```python
from build123d import *

# Parameters (mm, degrees)
SKETCH001_W     = 20
SKETCH001_H     = 84
PAD001_DEPTH    = 3
SKETCH002_W     = 20
SKETCH002_H     = 3
PAD002_DEPTH    = 10
SKETCH003_W     = 40
SKETCH003_H     = 8
SKETCH003_H_2   = 13
PAD003_DEPTH    = 3
FILLET_R        = 1
FILLET001_R     = 1
FILLET002_R     = 1
FILLET003_R     = 0.3
FILLET004_R     = 0.9
SKETCH009_W     = 10
SKETCH009_H     = 2
POCKET004_DEPTH = 5
POCKET005_DEPTH = 20


with BuildPart() as part:
    # Sketch001 → Pad001 (new body)
    with BuildSketch(Plane.XY):
        with Locations((0, -78.487457)):
            Rectangle(SKETCH001_W, SKETCH001_H)
    extrude(amount=PAD001_DEPTH)

    # Sketch002 → Pad002 (new body)
    with BuildSketch(Plane.XY.offset(3)):
        with Locations((0, -118.987457)):
            Rectangle(SKETCH002_W, SKETCH002_H)
        with Locations((0, -37.987457)):
            Rectangle(SKETCH002_W, SKETCH002_H)
    extrude(amount=PAD002_DEPTH)

    # Sketch003 → Pad003 (new body)
    with BuildSketch(Plane.XY.offset(13)):
        with Locations((0, -40.487457)):
            Rectangle(SKETCH003_W, SKETCH003_H)
        with Locations((0, -113.987457)):
            Rectangle(SKETCH003_W, SKETCH003_H_2)
    extrude(amount=PAD003_DEPTH)

    # Fillet
    fillet_edges = [part.edges().sort_by_distance(p)[0] for p in [
        (20, -113.987457, 16),
        (20, -113.987457, 13),
        (-20, -113.987457, 16),
        (0, -107.487457, 16),
        (0, -120.487457, 16),
        (-20, -113.987457, 13),
        (-15, -120.487457, 13),
        (15, -120.487457, 13),
    ]]
    fillet(fillet_edges, radius=FILLET_R)

    # Fillet001
    fillet001_edges = [part.edges().sort_by_distance(p)[0] for p in [
        (20, -40.487457, 16),
        (0, -44.487457, 16),
        (0, -36.487457, 16),
        (-20, -40.487457, 16),
        (-20, -40.487457, 13),
        (-15, -36.487457, 13),
        (15, -36.487457, 13),
        (20, -40.487457, 13),
        (0, -44.487457, 13),
    ]]
    fillet(fillet001_edges, radius=FILLET001_R)

    # Fillet002
    fillet002_edges = [part.edges().sort_by_distance(p)[0] for p in [
        (-10, -78.487457, 3),
        (-10, -117.487457, 8),
        (-10, -120.487457, 6.5),
        (-10, -78.487457, 0),
        (-10, -36.487457, 6.5),
        (10, -39.487457, 8),
        (10, -36.487457, 6.5),
        (10, -78.487457, 0),
        (10, -78.487457, 3),
        (10, -117.487457, 8),
        (10, -120.487457, 6.5),
    ]]
    fillet(fillet002_edges, radius=FILLET002_R)

    # Fillet003
    fillet003_edges = [part.edges().sort_by_distance(p)[0] for p in [
        (0, -39.487457, 3),
        (0, -117.487457, 3),
    ]]
    fillet(fillet003_edges, radius=FILLET003_R)

    # Fillet004
    fillet004_edges = [part.edges().sort_by_distance(p)[0] for p in [
        (0, -107.487457, 13),
    ]]
    fillet(fillet004_edges, radius=FILLET004_R)

    # Sketch009 → Pocket004 (cut)
    with BuildSketch(Plane(origin=(0, 0, 0), x_dir=(1, 0, 0), z_dir=(0, 0, -1))):
        with Locations((0, 40.487457)):
            Rectangle(SKETCH009_W, SKETCH009_H)
    extrude(amount=-POCKET004_DEPTH, mode=Mode.SUBTRACT)

    # Sketch012 → Pocket005 (cut)
    with BuildSketch(Plane(origin=(0, -36.487457, 0), x_dir=(-1, 0, 0), z_dir=(0, 1, 0))):
        with BuildLine():
            ThreePointArc((-4, 2), (-4.5, 1.5), (-4, 1))
            Line((-4, 1), (-2, 1))
            ThreePointArc((-2, 1), (-1.5, 1.5), (-2, 2))
            Line((-4, 2), (-2, 2))
        make_face()
        with BuildLine():
            ThreePointArc((2, 2), (1.5, 1.5), (2, 1))
            Line((2, 1), (4, 1))
            ThreePointArc((4, 1), (4.5, 1.5), (4, 2))
            Line((2, 2), (4, 2))
        make_face()
    extrude(amount=-POCKET005_DEPTH, mode=Mode.SUBTRACT)


solid = part.part
```
Input: part model. Units: mm. Frame: model coordinates. A direction names the side the tool comes from. Round coordinates to 2 decimals unless told otherwise and drop trailing zeros. Write each loop counter-clockwise with the first axis right and the second up, starting at its lowest first coordinate (ties: lowest second). Pieces come first, ordered by that corner, then holes. Notation, with made-up numbers: M -29.75,42 L 15.25,42 A33 cw 15.25,70 Z; hole C 36.25,-23 d5. An arc over 180 degrees is marked long. Write each question's results on one line, items separated by ' | '.
Q1. Line query: line 1 along Y through (x, z) = (-2, 12); line 2 along Z through (x, y) = (1.5, -103.5); line 3 along Z through (x, y) = (-10.5, -113). Output: solid intervals per line, ascending.
Results:
line 1: y = -120.49 to -117.49, -39.49 to -36.49 | line 2: z = 0 to 3 | line 3: z = 13 to 16
Q2. Section query C-C (y = -77). Return loops of the section in (x, z).
Results:
outline: M -10,1 A1 ccw -9,0 L 9,0 A1 ccw 10,1 L 10,2 A1 ccw 9,3 L -9,3 A1 ccw -10,2 Z
Q3. Section query A-A (z = 10). Return loops of the section in (x, y), and give its area (3 significant figures).
Results:
outline: M -10,-119.49 A1 ccw -9,-120.49 L 9,-120.49 A1 ccw 10,-119.49 L 10,-118.49 A1 ccw 9,-117.49 L -9,-117.49 A1 ccw -10,-118.49 Z; M -10,-39.49 L 9,-39.49 A1 ccw 10,-38.49 L 10,-37.49 A1 ccw 9,-36.49 L -9,-36.49 A1 ccw -10,-37.49 Z | area: 118 mm^2
Q4. Draft query along Z for faces 6 (the face through (-3, -49, 1)), 7 (the face through (0, -78, 0)), 8 (the face through (5, -40, 2)). Return one class per face: released by +Z, released by -Z, zero draft, split by the parting line, or undercut.
Results:
face 6: undercut | face 7: released by -Z | face 8: zero draft
Q5. Section query B-B (x = -11). Return loops of the section in (y, z).
Results:
outline: M -120.49,14 A1 ccw -119.49,13 L -108.39,13 A0.9 ccw -107.49,13.9 L -107.49,15 A1 ccw -108.49,16 L -119.49,16 A1 ccw -120.49,15 Z; M -44.49,14 A1 ccw -43.49,13 L -37.49,13 A1 ccw -36.49,14 L -36.49,15 A1 ccw -37.49,16 L -43.49,16 A1 ccw -44.49,15 Z
Q6. Access query for faces 1 (the face through (3, -49, 2)), 2 (the face through (-5, -40, 2)), 3 (the face through (0, -78, 3)), 4 (the face through (0, -36.487, 7)), 5 (the face through (-1, -39.487, 6)). Directions: +Z, -Z, +X, -X, +Y, -Y. A direction counts if a zero-diameter tool reaches every point of the face in a straight line with its end or side. Return the directions, or none.
Results:
face 1: +Y | face 2: -Z | face 3: +X, -X | face 4: +Z, -Z, +X, -X, +Y | face 5: none
Q7. Pin query (flat end, axial travel): P1, Ø4, axis at x = -7, y = -48, coming from the +Z side; P2, Ø2, axis at y = -40, z = 1, coming from the -X side. Return the tip coordinate at first contact, or that it passes through.
Results:
P1: stops at z = 3 | P2: stops at x = -10
